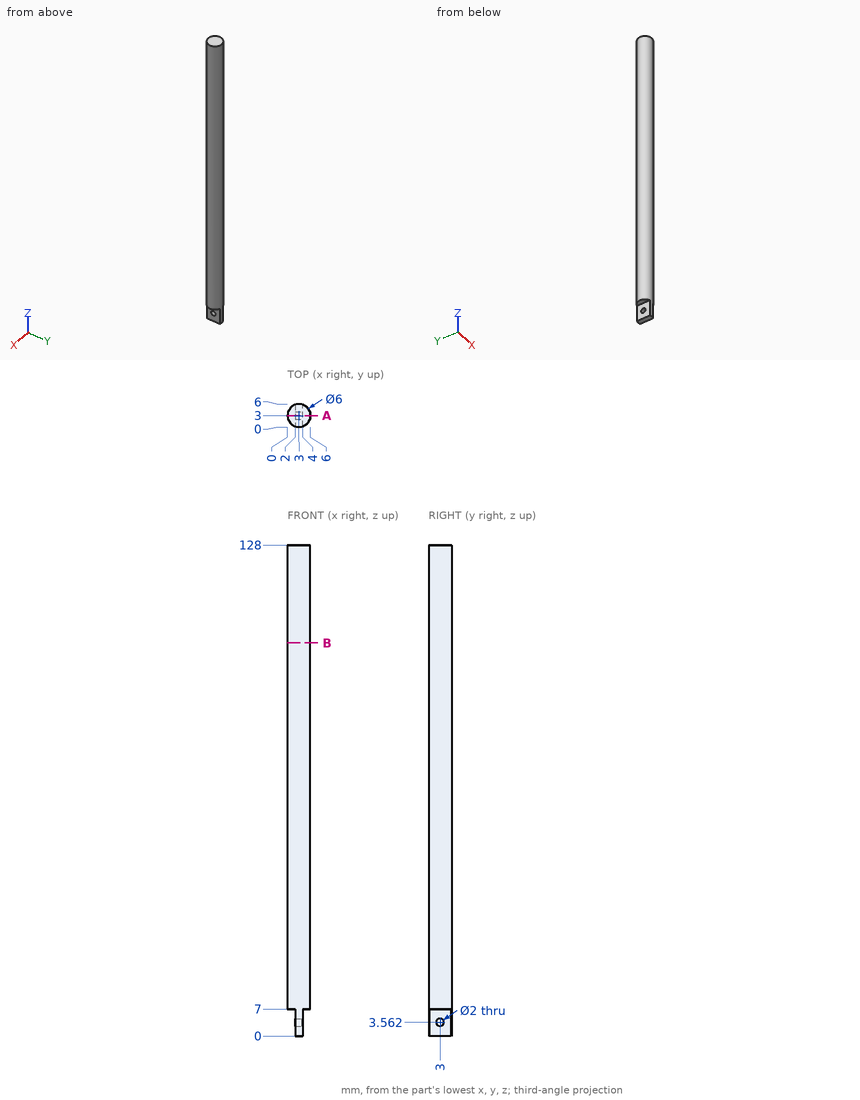
Can you work these out from the drawing? Everything is in mm from the part's minimum corner. Round coordinates to 2 decimals unless told otherwise and drop trailing zeros. Loops run counter-clockwise (first coordinate to the right, second up) from the corner with the lowest first, then second, coordinate; pieces in that order, holes last. Notation, with made-up numbers: (14.5, -40) - (53.5, -40) arc R23 cw to (53.5, -2) - close; hole circle Ø3 at (42, -2). An arc over 180 degrees is marked (long way). One line per question, with ' | ' between items. Start each with the question number.
Q1. Will these pins go through, and if not, where does the flat tip stop? pin 1 (2.5 mm diameter, centred on y = 3, z = 3.56, fed in from -X); pin 2 (1.7 mm diameter, centred on y = 2, z = 3.5, fed in from +X); pin 3 (1 mm diameter, centred on x = 4, z = 47.5, fed in from -Y).
Q2. I want a section at B-B (z = 102.5). Write out the boundary of the cut face in (x, y).
Q3. Please list where these lines run through material, in increasing order: line 1 (Z direction, x = 3.3, y = 3); line 2 (Z direction, x = 5.3, y = 3.35); line 3 (Y direction, x = 2.8, z = 96). Write a range as [from, to].
Q4. I want a section at A-A (y = 3). Write out the boundary of the cut face in (x, z), then the cut area to 3 significant figures.
Response values:
1) pin 1: stops at x = 2 | pin 2: stops at x = 4 | pin 3: stops at y = 0.04
2) outline: circle Ø6 at (3, 3)
3) line 1: z = [0, 2.56], [4.56, 128] | line 2: z = [7, 128] | line 3: y = [0.01, 5.99]
4) outline: (0, 7) - (2, 7) - (2, 4.56) - (4, 4.56) - (4, 7) - (6, 7) - (6, 128) - (0, 128) - close; (2, 0) - (4, 0) - (4, 2.56) - (2, 2.56) - close | area: 736 mm²
